Verification items for this drawing (mm, ordinates from the low corner). A direction names the side the tool comes from. Round coordinates to 2 decimals unless told otherwise and drop trailing zeros. Order: outer loops, then holes, each group sorted by start corner. A loop starts at its lowest first (then second) coordinate and runs counter-clockwise, first axis right, second up. Notation, with made-up numbers: M -32.5,19 L -6.5,19 A24 ccw -6.5,32 Z; hole C 39.25,-4.5 d4. An arc over 180 degrees is marked long. One line per item, written item: value. Start each with the question number.
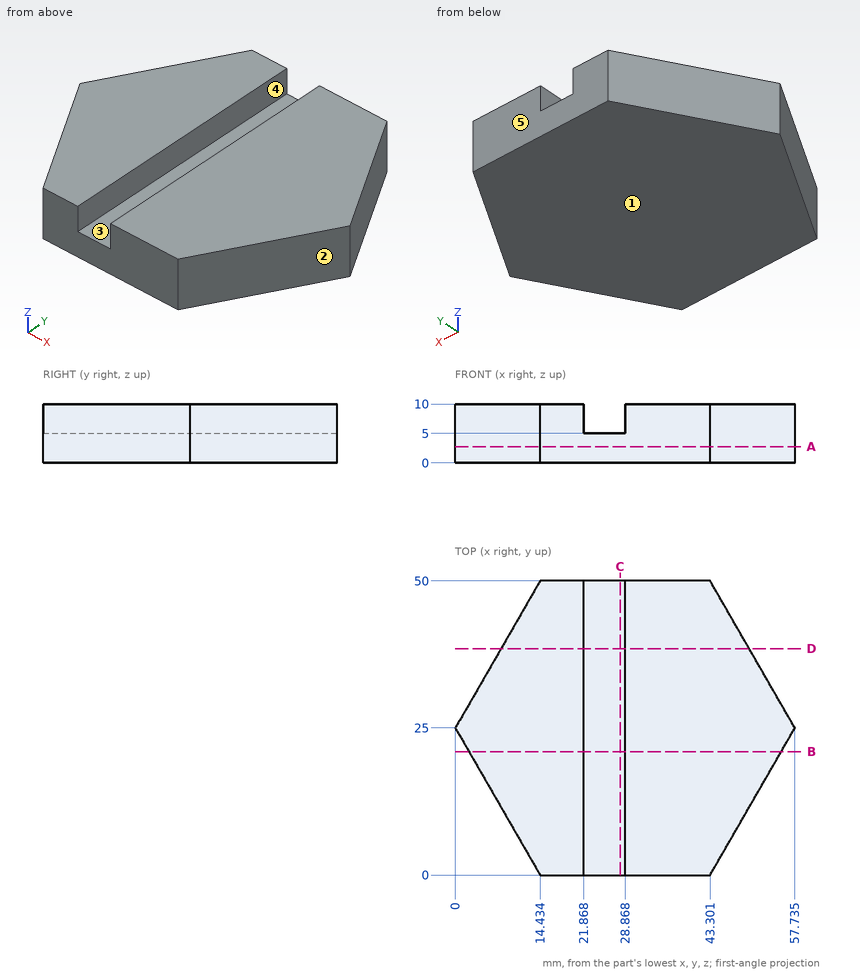
1. Scan lines: line 1 along Z through (x, y) = (22.5, 44); line 2 along X through (y, z) = (18, 6) (1 decimal); line 3 along X through (y, z) = (45.5, 7) (1 decimal). Record each from-to range of solid material in increasing order.
2. Section check D-D (y = 38.5). Record the cut outline in (x, z) (1 decimal).
3. Depth check by flat-ended pin: pin 1 (5.5 mm diameter, centred on y = 31.5, z = 8, fed in from +X); pin 2 (1 mm diameter, centred on y = 13, z = 7, fed in from +X) (1 decimal); pin 3 (4 mm diameter, centred on y = 30.5, z = 7.5, fed in from -X). Enter the tip coordinate at first touch or a pass-through.
4. Section check A-A (z = 2.75). Record the cut outline in (x, y) (1 decimal), and give its area (4 significant figures).
5. Section check C-C (x = 28). Record the cut outline in (y, z).
6. Section check B-B (y = 21). Record the cut outline in (x, z) (1 decimal), and give its area (3 significant figures).
7. Draft check along X on the marked faces 1, 2 and 3. Enter one of: released by +X, released by -X, zero draft, split by the parting line, or undercut.
8. Tool access check on the marked faces 4 and 5. Record the directions out of +Z, -Z, +X, -X, +Y, -Y that give a thin tool (end or side, any length) a straight path to the whole face; none if there is none.
Geometry check:
1. line 1: z = 0 to 5
1. line 2: x = 4 to 21.9, 28.9 to 53.7
1. line 3: x = 11.8 to 21.9, 28.9 to 45.9
2. outline: M 7.8,0 L 49.9,0 L 49.9,10 L 28.9,10 L 28.9,5 L 21.9,5 L 21.9,10 L 7.8,10 Z
3. pin 1: stops at x = 55.57
3. pin 2: stops at x = 51.1
3. pin 3: stops at x = 2.02
4. outline: M 0,25 L 14.4,0 L 43.3,0 L 57.7,25 L 43.3,50 L 14.4,50 Z
4. area: 2,165 mm²
5. outline: M 0,0 L 50,0 L 50,5 L 0,5 Z
6. outline: M 2.3,0 L 55.4,0 L 55.4,10 L 28.9,10 L 28.9,5 L 21.9,5 L 21.9,10 L 2.3,10 Z
6. area: 496 mm²
7. face 1: zero draft
7. face 2: released by +X
7. face 3: undercut
8. face 4: +Z, +Y, -Y
8. face 5: +Z, -Z, +X, -X, +Y
